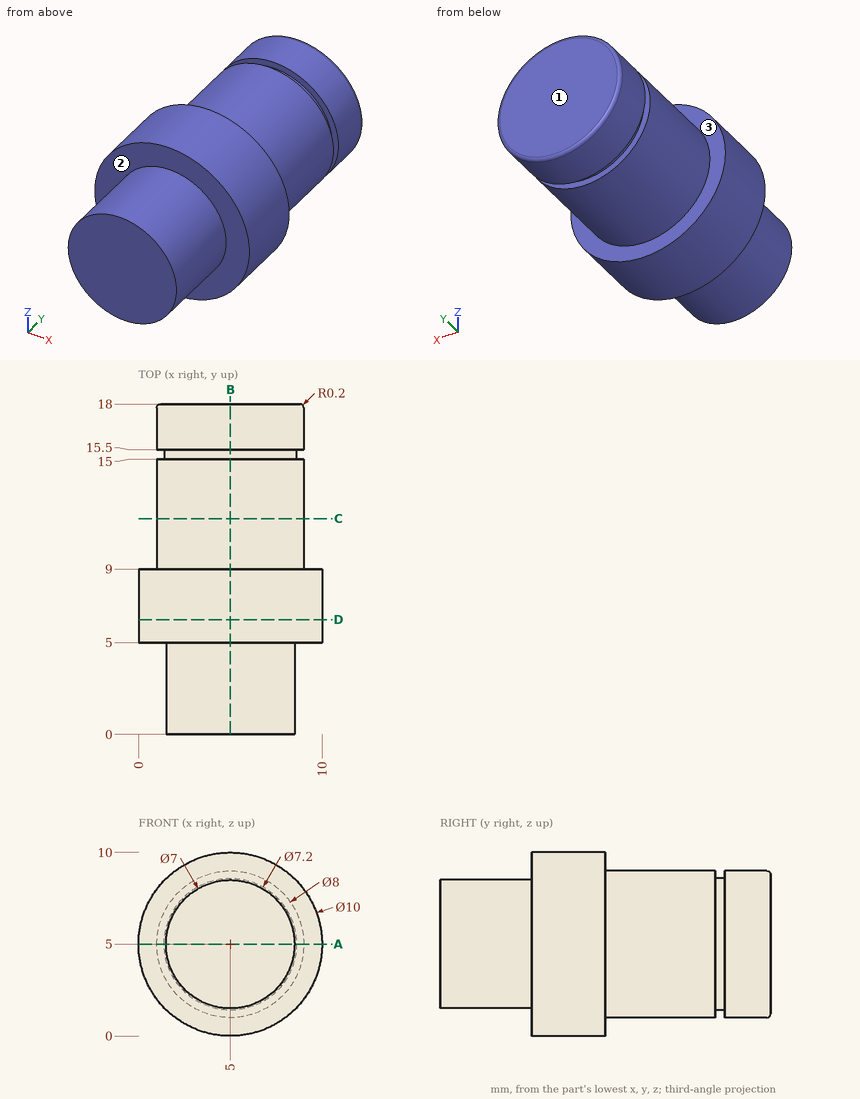
Geometry: see drawing. Coordinates: mm, zero at the bounding-box minimum. A direction names the side the tool comes from. Coordinates: 2 decimals unless noted, no trailing zeros. Order: outer loops, then holes, each group sorted by start corner. A loop starts at its lowest first (then second) coordinate and runs counter-clockwise, first axis right, second up. Notation, with made-up numbers: M -35,23.25 L -29,23.25 A26 cw -29,47.25 Z; hole C 83.25,-39 d9. An arc over 180 degrees is marked long. Answer as CSV lines item,"result".
1. Access query for the marked faces 1, 2 and 3. Directions: +Z, -Z, +X, -X, +Y, -Y. A direction counts if a zero-diameter tool reaches every point of the face in a straight line with its end or side. Return the directions, or none.
Reported:
face 1,"+Z, -Z, +X, -X, +Y"
face 2,"-Y"
face 3,"+Y"
2. First-contact query: P1, Ø3, axis at y = 6, z = 8.5, coming from the +X side; P2, Ø2, axis at y = 13.5, z = 7, coming from the +X side; P3, Ø4, axis at y = 12, z = 5.5, coming from the +X side; P4, Ø6, axis at y = 7, z = 8, coming from the -X side. Flat tips, straight axial feed; report the tip coordinate or a pass-through.
Reported:
P1,"x = 9.58"
P2,"x = 8.87"
P3,"x = 9"
P4,"x = 0"
3. Material intervals for line 1 (Y direction, x = 2.75, z = 0.75); line 2 (Z direction, x = 5, y = 9.25); line 3 (X direction, y = 14, z = 6.75), sorted ascending. Write a range as from..to.
Reported:
line 1,"5..9"
line 2,"1..9"
line 3,"1.4..8.6"
4. Section D-D (y = 6.25). Return the cut outline in (x, z).
Reported:
outline,"C 5,5 d10"
5. Section C-C (y = 11.75). Return the cut outline in (x, z).
Reported:
outline,"C 5,5 d8"
6. Section B-B (x = 5). Return the cut outline in (y, z), then the cut area to 3 significant figures.
Reported:
outline,"M 0,1.5 L 5,1.5 L 5,0 L 9,0 L 9,1 L 15,1 L 15,1.4 L 15.5,1.4 L 15.5,1 L 17.8,1 A0.2 ccw 18,1.2 L 18,8.8 A0.2 ccw 17.8,9 L 15.5,9 L 15.5,8.6 L 15,8.6 L 15,9 L 9,9 L 9,10 L 5,10 L 5,8.5 L 0,8.5 Z"
area,"147 mm2"
7. Section A-A (z = 5). Return the cut outline in (x, y).
Reported:
outline,"M 0,5 L 1.5,5 L 1.5,0 L 8.5,0 L 8.5,5 L 10,5 L 10,9 L 9,9 L 9,15 L 8.6,15 L 8.6,15.5 L 9,15.5 L 9,17.8 A0.2 ccw 8.8,18 L 1.2,18 A0.2 ccw 1,17.8 L 1,15.5 L 1.4,15.5 L 1.4,15 L 1,15 L 1,9 L 0,9 Z"
